Solid Edge part; units mm, degrees
sketch "Sketch1" plane through (0, 0, 0) normal (0, 0, 1) x (1, 0, 0)
  circle A0 centre (0, 0) radius 54.65
extrude "Protrusion1" add sketch "Sketch1" along normal blind 14
sketch "Sketch2" plane through (0, 0, 0) normal (0, 0, 1) x (1, 0, 0)
  line L0 (-52.5511, 15) -> (-52.5511, -15)
extrude "Cutout1" cut sketch "Sketch2" along normal through all material side at (-52.6011, 0, 0)
sketch "Sketch3" plane through (-52.5511, 0, 6) normal (-1, 0, 0) x (0, -1, 0)
  line L0 (14.4, 5) -> (-14.4, 5)
  line L1 (-14.4, 5) -> (-14.4, -3)
  line L2 (-14.4, -3) -> (14.4, -3)
  line L3 (14.4, -3) -> (14.4, 5)
extrude "Extrusionsausschnitt_5" cut sketch "Sketch3" against normal blind 30
sketch "Sketch4" plane through (-24.581, 0, 3) normal (0, 0, 1) x (0, -1, 0)
  line L0 (-7.5, -7.9701) -> (-7.5, -22.9701)
  line L1 (-7.5, -22.9701) -> (-11, -22.9701)
  line L2 (-11, -22.9701) -> (-11, -7.9701)
  line L3 (-11, -7.9701) -> (-7.5, -7.9701)
extrude "Cutout2" cut sketch "Sketch4" against normal through all
mirror "Mirror1" about plane through (0, 0, 0) normal (0, -1, 0) of "Cutout2"
pattern_circular "Pattern1" count 3 over 360 about axis through (0, 0, 0) along (0, 0, -1) of "Mirror1", "Cutout2", "Extrusionsausschnitt_5", "Cutout1"
hole "Bohrung_3" at (12, 0, 0) direction (0, 0, 1) diameter 3.2 end through all
hole "Hole1" at (24, 0, 0) direction (0, 0, 1) diameter 3.2 end through all
hole "Bohrung_5" at (-12, 0, 0) direction (0, 0, 1) diameter 3.2 end through all
hole "Bohrung_6" at (-11, 32, 0) direction (0, 0, 1) diameter 2.7 end through all
hole "Hole2" at (-11, -32, 0) direction (0, 0, 1) diameter 2.7 end through all
hole "Bohrung_8" at (-12, 0, 0) direction (0, 0, 1) diameter 7 depth 1
hole "Hole3" at (12, 0, 0) direction (0, 0, 1) diameter 7 depth 1
hole "Hole4" at (24, 0, 0) direction (0, 0, 1) diameter 7 depth 1
properties material "PLA"
Check sheet for the modelled part. Datum: model origin and axes. Units: mm. A direction names the side the tool comes from. Give positions to 0.01 mm unless a question says otherwise; leave off trailing zeros. Write each loop counter-clockwise with the first axis right and the second up, starting at its lowest first coordinate (ties: lowest second). Pieces come first, ordered by that corner, then holes. Notation, with made-up numbers: (6, 83) -> (29, 83) arc R26 ccw to (29, 104) -> close; hole circle Ø6 at (-32, 15.25). An arc over 180 degrees is marked (long way). One line per item, written item: value. Start each with the question number.
Item 1: Section check A-A on z = 8.75. Record the cut outline in (x, y).
Item 2: Section check B-B on y = 0. State how many separate pieces and enclosed holes the cut face has, then the cut area to 3 significant figures.
Item 3: Gauge pin test, flat ends, axial feed: pin 1 (1.5 mm diameter, centred on y = 28, z = 4.5, fed in from -X); pin 2 (2 mm diameter, centred on y = -42, z = 8.5, fed in from -X); pin 3 (2 mm diameter, centred on x = -11, y = 32, fed in from +Z); pin 4 (3.5 mm diameter, centred on y = -10, z = 1.5, fed in from +X). Record the tip position at first contact, or that the pin passes through.
Item 4: Tool access check on faces 4 (the flat face through (24.31, 23.55, 1.52)), 5 (the flat face through (26.457, 45.406, 2.235)). Record the directions out of +Z, -Z, +X, -X, +Y, -Y that give a thin tool (end or side, any length) a straight path to the whole face; none if there is none.
Item 5: Draft check along X on faces 1 (the flat face through (26.457, -45.406, 2.235)), 2 (the flat face through (-22.551, 0, 7)), 3 (the cylindrical face through (13.586, -0.208, 7.409)). Enter one of: +X half, -X half, draft (parallel to the pull), parting line (faces both ways), or undercut.
Item 6: Section check D-D on y = 43.5. Record the cut outline in (x, z).
Item 7: Material ranges on probe 1 along Z at (x, y) = (30.5, 41); probe 2 along Y at (x, z) = (1.5, 9.5); probe 3 along X at (y, z) = (0, 11.5), recorded low to high. Write a range as from..to.
Item 8: Section check C-C on x = 12. Record the cut outline in (y, z), then the cut area to 3 significant figures.
Results list:
1. outline: (-52.55, -15) arc R54.65 ccw to (13.29, -53.01) -> (13.8, -52.71) -> (-1.2, -26.73) -> (23.75, -12.33) -> (38.75, -38.31) -> (39.27, -38.01) arc R54.65 ccw to (39.27, 38.01) -> (38.75, 38.31) -> (23.75, 12.33) -> (-1.2, 26.73) -> (13.8, 52.71) -> (13.29, 53.01) arc R54.65 ccw to (-52.55, 15) -> (-52.55, 14.4) -> (-22.55, 14.4) -> (-22.55, -14.4) -> (-52.55, -14.4) -> close; hole circle Ø3.2 at (-12, 0); hole circle Ø2.7 at (-11, -32); hole circle Ø2.7 at (-11, 32); hole circle Ø3.2 at (12, 0); hole circle Ø3.2 at (24, 0)
2. separate pieces: 4
2. enclosed holes: 0
2. area: 1,120 mm²
3. pin 1: x = -47.37
3. pin 2: x = -36.13
3. pin 3: through
3. pin 4: x = 54.02
4. face 4: -Z
4. face 5: +Z, -Z, +X, +Y
5. face 1: +X half
5. face 2: -X half
5. face 3: undercut
6. outline: (-33.08, 0) -> (12.41, 0) -> (12.41, 3) -> (8.49, 3) -> (8.49, 11) -> (29.76, 11) -> (29.76, 14) -> (-33.08, 14) -> close; (16.45, 0) -> (29.76, 0) -> (29.76, 3) -> (16.45, 3) -> close
7. probe 1: 0..3, 11..14
7. probe 2: -54.63..-31.4, -25.17..25.17, 31.4..54.63
7. probe 3: -52.55..-13.6, -10.4..10.4, 13.6..22.4, 25.6..54.65
8. outline: (-53.32, 0) -> (-42.78, 0) -> (-42.78, 3) -> (-49.58, 3) -> (-49.58, 11) -> (-19.11, 11) -> (-19.11, 3) -> (-35.78, 3) -> (-35.78, 0) -> (-3.5, 0) -> (-3.5, 1) -> (-1.6, 1) -> (-1.6, 14) -> (-53.32, 14) -> close; (1.6, 1) -> (3.5, 1) -> (3.5, 0) -> (35.78, 0) -> (35.78, 3) -> (19.11, 3) -> (19.11, 11) -> (49.58, 11) -> (49.58, 3) -> (42.78, 3) -> (42.78, 0) -> (53.32, 0) -> (53.32, 14) -> (1.6, 14) -> close
8. area: 915 mm²
